from build123d import *

# Parameters (mm, degrees)
SKETCH1_R           = 3.57
BOSS_EXTRUDE1_DEPTH = 5


with BuildPart() as part:
    # Sketch1 → Boss-Extrude1 (new body)
    with BuildSketch(Plane(origin=(0, 0, 0), x_dir=(0, 0, -1), z_dir=(1, 0, 0))):
        with BuildLine():
            Line((-34.292652671, 6.101206192), (-25.106065934, 9.812828159))
            ThreePointArc((-25.106065934, 9.812828159), (-21.36, 10.540989614), (-17.613934066, 9.812828159))
            Line((-17.613934066, 9.812828159), (-8.427347329, 6.101206192))
            ThreePointArc((-8.427347329, 6.101206192), (-5.123042901, 5.382807164), (-1.768225144, 5.806744341))
            ThreePointArc((-1.768225144, 5.806744341), (5.628005997, -2.273862022), (-5.305658284, -2.948709917))
            ThreePointArc((-5.305658284, -2.948709917), (-7.424420711, -0.313302797), (-10.300380296, 1.465286919))
            Line((-10.300380296, 1.465286919), (-17.613934066, 4.420154446))
            ThreePointArc((-17.613934066, 4.420154446), (-21.36, 5.1483159), (-25.106065934, 4.420154446))
            Line((-25.106065934, 4.420154446), (-32.419619704, 1.465286919))
            ThreePointArc((-32.419619704, 1.465286919), (-35.295579289, -0.313302797), (-37.414341716, -2.948709917))
            ThreePointArc((-37.414341716, -2.948709917), (-48.348005997, -2.273862022), (-40.951774856, 5.806744341))
            ThreePointArc((-40.951774856, 5.806744341), (-37.596957099, 5.382807164), (-34.292652671, 6.101206192))
        make_face()
        Circle(SKETCH1_R, mode=Mode.SUBTRACT)
        with Locations((-42.72, 0)):
            Circle(SKETCH1_R, mode=Mode.SUBTRACT)
    extrude(amount=BOSS_EXTRUDE1_DEPTH)


solid = part.part
The listing builds one solid part. Answer for the finished solid, in the listing's coordinates (mm). A direction names the side the tool comes from. Give positions to 0.01 mm unless a question says otherwise; leave off trailing zeros. Order: outer loops, then holes, each group sorted by start corner. A loop starts at its lowest first (then second) coordinate and runs counter-clockwise, first axis right, second up. Notation, with made-up numbers: (39.25, 52) -> (57.25, 52) arc R21 ccw to (57.25, 87) -> close; hole circle Ø9 at (18.25, -17.5). An arc over 180 degrees is marked (long way). Put each result on its own line as item: value.
Item 1: For a pull along Y with two mould halves and no side action, classify faces 1 (the face through (2.465, 1.072, -3.405)), 2 (the face through (2.465, 2.963, 28.712)), 3 (the face through (2.46, 7.98, 13.08)) as released by +Y, released by -Y, zero draft, split by the parting line, or undercut.
Established:
face 1: undercut
face 2: released by -Y
face 3: released by +Y
Item 2: A cutting plane is placed at C-C on x = 3.35. Give the vertices of the cut face in (y, z).
Established:
outline: (-2.95, 5.31) arc R6.07 ccw (long way) to (5.81, 1.77) arc R10 cw to (6.1, 8.43) -> (9.81, 17.61) arc R10 ccw to (9.81, 25.11) -> (6.1, 34.29) arc R10 cw to (5.81, 40.95) arc R6.07 ccw (long way) to (-2.95, 37.41) arc R10 cw to (1.47, 32.42) -> (4.42, 25.11) arc R10 cw to (4.42, 17.61) -> (1.47, 10.3) arc R10 cw to start; hole circle Ø7.14 at (0, 0); hole circle Ø7.14 at (0, 42.72)
Item 3: Given P1, Ø1, axis at y = 2.5, z = 16, coming from the -X side; P2, Ø2, axis at x = 4, z = 26.5, coming from the +Y side, each flat-ended and moving along its own axis, determine where each tip first touches the part or whether it passes through.
Established:
P1: passes through
P2: stops at y = 9.65
Item 4: For faces 4 (the face through (2.465, -2.095, -5.697)), 5 (the face through (2.465, 2.922, 13.906)), determine the directions among +Z, -Z, +X, -X, +Y, -Y from which every point of the face is accessible in a straight line to the end or side of a thin tool.
Established:
face 4: +X, -X
face 5: +X, -X, -Y
Item 5: A cutting plane is placed at B-B on y = 0. Give the vertices of the cut face in (x, z), plus the area to 3 significant figures.
Established:
outline: (0, -6.07) -> (5, -6.07) -> (5, -3.57) -> (0, -3.57) -> close; (0, 3.57) -> (5, 3.57) -> (5, 7.8) -> (0, 7.8) -> close; (0, 34.92) -> (5, 34.92) -> (5, 39.15) -> (0, 39.15) -> close; (0, 46.29) -> (5, 46.29) -> (5, 48.79) -> (0, 48.79) -> close
area: 67.3 mm^2
Item 6: A cutting plane is placed at A-A on z = 0. Give the vertices of the cut face in (x, y).
Established:
outline: (0, -6.07) -> (5, -6.07) -> (5, -3.57) -> (0, -3.57) -> close; (0, 3.57) -> (5, 3.57) -> (5, 6.07) -> (0, 6.07) -> close
Item 7: A cutting plane is placed at D-D on z = 45.5. Give the vertices of the cut face in (x, y), plus the area to 3 significant figures.
Established:
outline: (0, -5.4) -> (5, -5.4) -> (5, -2.24) -> (0, -2.24) -> close; (0, 2.24) -> (5, 2.24) -> (5, 5.4) -> (0, 5.4) -> close
area: 31.6 mm^2
Item 8: Straight lines are drawn through the part: line 1 (Z direction, x = 3.3, y = -3); line 2 (Y direction, x = 2.3, z = 0); line 3 (Z direction, x = 3.05, y = 3.25). For each, find the intervals that lie inside material, in ascending order.
Established:
line 1: z = -5.28 to -1.94, 1.94 to 5.28, 37.44 to 40.78, 44.66 to 48
line 2: y = -6.07 to -3.57, 3.57 to 6.07
line 3: z = -5.13 to -1.48, 1.48 to 14.72, 28 to 41.24, 44.2 to 47.85
